Design review of the part shown in the three views and the two pictorial views. Dimensions are in mm from the part's minimum x, y and z. A direction names the side the tool comes from. Coordinates: 2 decimals unless noted, no trailing zeros. Loops run counter-clockwise (first coordinate to the right, second up) from the corner with the lowest first, then second, coordinate; pieces in that order, holes last.
Q1. For P1, Ø1.8, axis at x = 15, z = 3.5, coming from the -Y side; P2, Ø1.5, axis at x = 8, y = 16, coming from the +Z side; P3, Ø1.6, axis at y = 17, z = 0.5, coming from the -X side; P4, Ø2, axis at y = 16.5, z = 1.5, coming from the +X side, all flat-tipped, find the tip position at first contact; note any pin that passes through.
Q2. Add section C-C on y = 10.5. Give the boundary of the cut face in (x, z).
Q3. Add section B-B on x = 17. Give the boundary of the cut face in (y, z), and give its area (3 significant figures).
Q4. Add section D-D on z = 3.4. Give the boundary of the cut face in (x, y).
Q5. Machinability: for the marked faces 1, 2, 3 and 4, which of the approach directions +Z, -Z, +X, -X, +Y, -Y give a long, thin tool a straight path to every point of the face, cutting with its end or side? Answer none if there is none.
Q6. Add section A-A on z = 1.6. Give the boundary of the cut face in (x, y), and give its area (3 significant figures).
Q7. Wall thickness on probe 1 along Z at (x, y) = (3.5, 8.75); probe 2 along Y at (x, z) = (17, 4.2); probe 3 along X at (y, z) = (4.5, 0.5): over which ranges is each line inside the solid? List them lowest first.
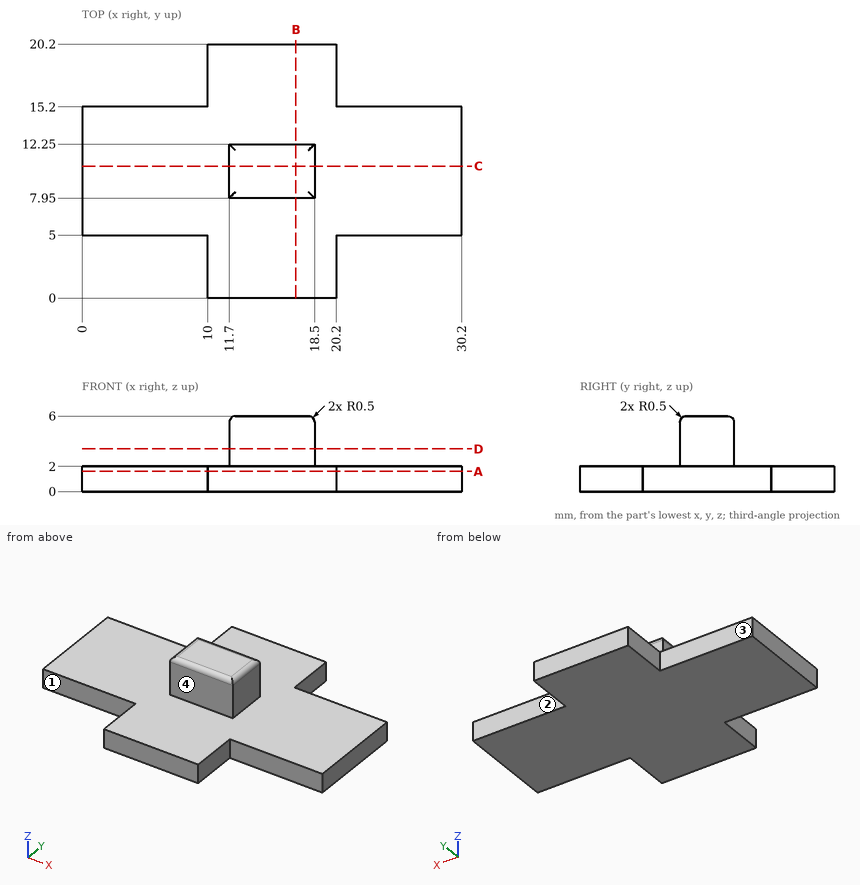
Entries:
1. P1: stops at y = 7.95
1. P2: passes through
1. P3: stops at x = 10
1. P4: stops at x = 20.2
2. outline: (0, 0) - (30.2, 0) - (30.2, 2) - (18.5, 2) - (18.5, 5.5) arc R0.5 ccw to (18, 6) - (12.2, 6) arc R0.5 ccw to (11.7, 5.5) - (11.7, 2) - (0, 2) - close
3. outline: (0, 0) - (20.2, 0) - (20.2, 2) - (12.25, 2) - (12.25, 5.5) arc R0.5 ccw to (11.75, 6) - (8.45, 6) arc R0.5 ccw to (7.95, 5.5) - (7.95, 2) - (0, 2) - close
3. area: 57.5 mm2
4. outline: (11.7, 7.95) - (18.5, 7.95) - (18.5, 12.25) - (11.7, 12.25) - close
5. face 1: +Z, -Z, -X, -Y
5. face 2: +Z, -Z, +X, +Y
5. face 3: +Z, -Z, -X, +Y
5. face 4: +Z, +X, -X, -Y
6. outline: (0, 5) - (10, 5) - (10, 0) - (20.2, 0) - (20.2, 5) - (30.2, 5) - (30.2, 15.2) - (20.2, 15.2) - (20.2, 20.2) - (10, 20.2) - (10, 15.2) - (0, 15.2) - close
6. area: 410 mm2
7. probe 1: z = 0 to 2
7. probe 2: y = 7.95 to 12.25
7. probe 3: x = 10 to 20.2
